The figure shows three views and two pictorial views of one solid part (mm, origin at its lowest corner). Answer the questions. Coordinates: 2 decimals unless noted, no trailing zeros. Write each loop counter-clockwise with the first axis right and the second up, starting at its lowest first coordinate (ties: lowest second). Pieces come first, ordered by that corner, then holes.
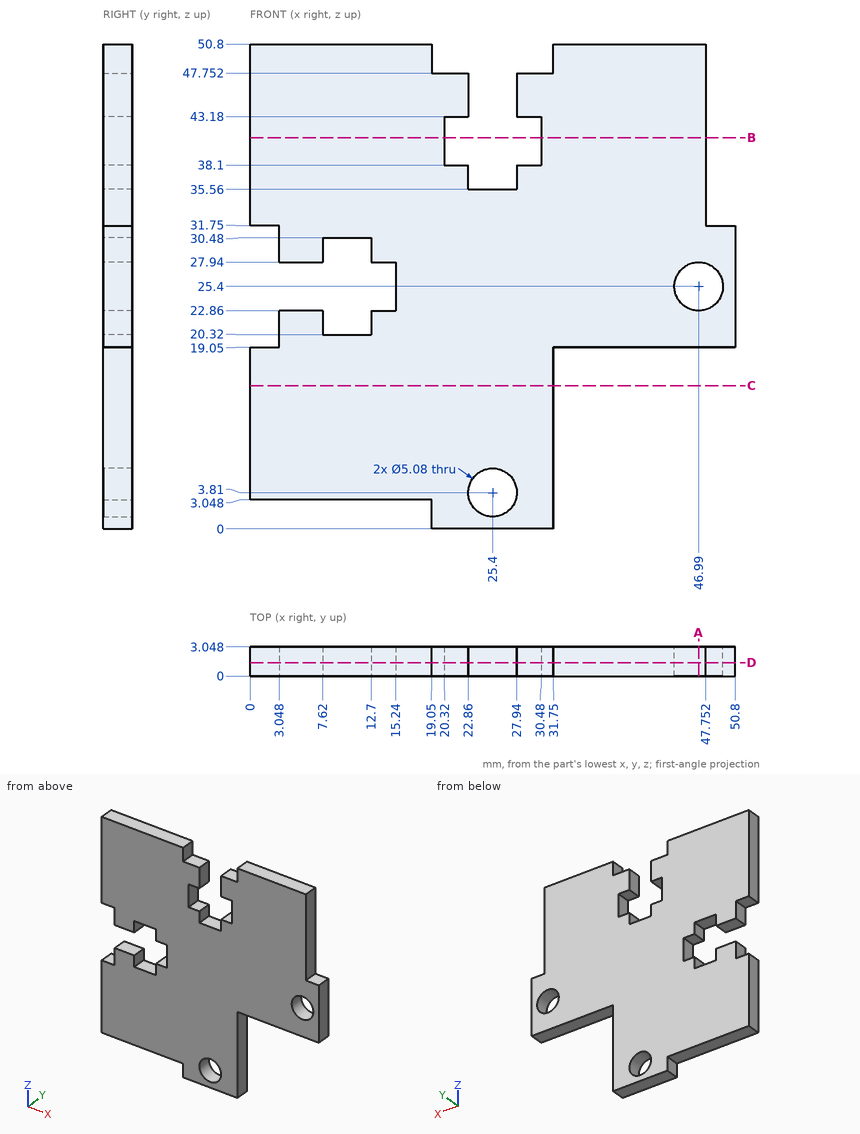
1. Flat-ended cylindrical pins translate along their axes: P1, Ø1.5, axis at y = 1, z = 20, coming from the -X side; P2, Ø1.5, axis at y = 1, z = 40, coming from the +X side; P3, Ø1.5, axis at x = 9.5, y = 2, coming from the -Z side. Find the tip coordinate at first contact, or state that the pin passes through.
Results found:
P1: stops at x = 3.05
P2: stops at x = 47.75
P3: stops at z = 3.05
2. Section A-A on x = 46.99 is taken. Give the vertices of the cut face in (y, z).
Results found:
outline: (0, 19.05) - (3.05, 19.05) - (3.05, 22.86) - (0, 22.86) - close; (0, 27.94) - (3.05, 27.94) - (3.05, 50.8) - (0, 50.8) - close
3. Section D-D on y = 1.4 is taken. State how many separate pieces and enclosed holes the cut face has, then the cut area to 3 significant figures.
Results found:
separate pieces: 1
enclosed holes: 2
area: 1,810 mm2
4. Section B-B on z = 41 is taken. Give the vertices of the cut face in (x, y), then the cut area to 3 significant figures.
Results found:
outline: (0, 0) - (20.32, 0) - (20.32, 3.05) - (0, 3.05) - close; (30.48, 0) - (47.75, 0) - (47.75, 3.05) - (30.48, 3.05) - close
area: 115 mm2
5. Section C-C on z = 15 is taken. Give the vertices of the cut face in (x, y), then the cut area to 3 significant figures.
Results found:
outline: (0, 0) - (31.75, 0) - (31.75, 3.05) - (0, 3.05) - close
area: 96.8 mm2
6. Find the intervals of material crossed by L1, parallel to X at y = 2.25, z = 44; L2, parallel to X at y = 0.7, z = 25.4; L3, parallel to Z at x = 5, y = 2.65, in increasing order.
Results found:
L1: x = 0 to 22.86, 27.94 to 47.75
L2: x = 15.24 to 44.45, 49.53 to 50.8
L3: z = 3.05 to 22.86, 27.94 to 50.8
